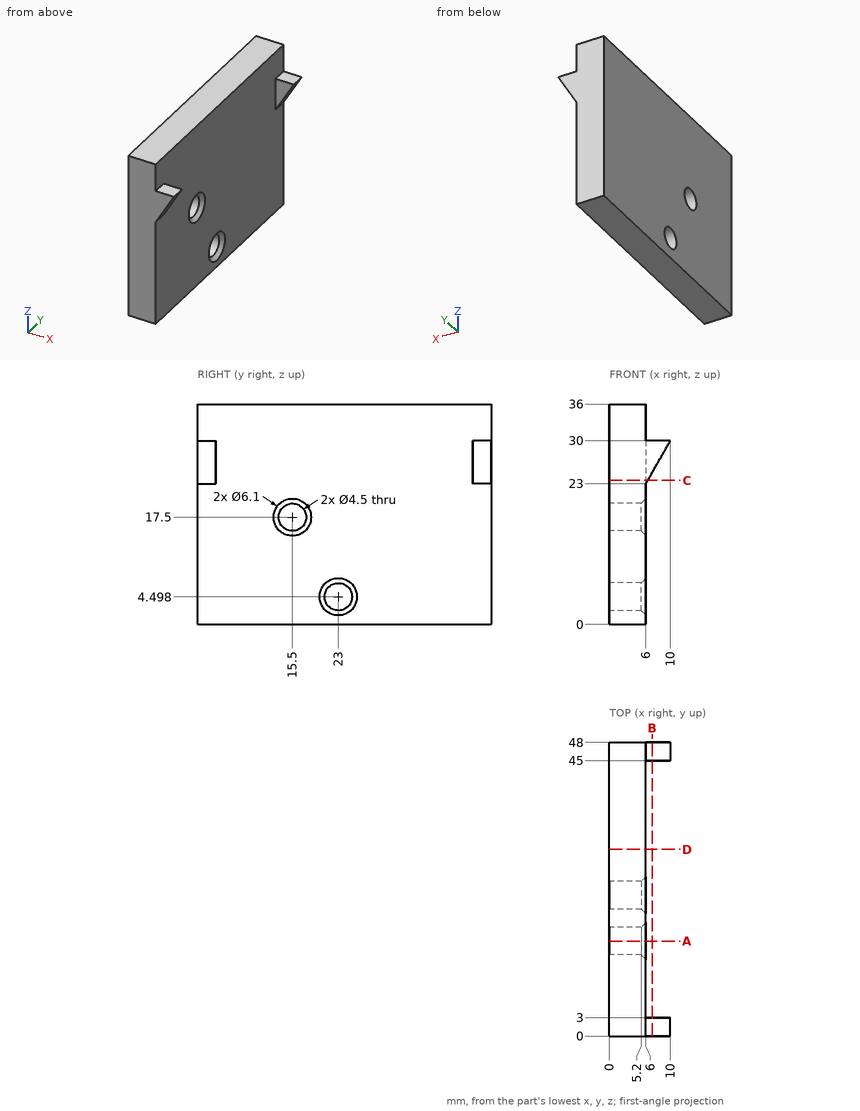
Input: dimensioned drawing with shaded views. Units: mm. Origin: part minimum x, y, z. Give positions to 0.01 mm unless a question says otherwise; leave off trailing zeros. Loops run counter-clockwise (first coordinate to the right, second up) from the corner with the lowest first, then second, coordinate; pieces in that order, holes last. Notation, with made-up numbers: (2.5, 26) -> (16.5, 26) arc R24 cw to (16.5, 54) -> close; hole circle Ø8 at (78.5, 4). An arc over 180 degrees is marked (long way). Use a Markdown table: item, result. Add a question column.
1) First-contact query: pin 1 (11 mm diameter, centred on y = 34, z = 21, fed in from +X); pin 2 (5 mm diameter, centred on x = 9, y = 8.5, fed in from +Z); pin 3 (0.9 mm diameter, centred on x = 7, y = 2, fed in from +Z). Flat tips, straight axial feed; report the tip coordinate or a pass-through.
2) Line query: line 1 along Z through (x, y) = (3.25, 23); line 2 along Y through (x, z) = (2.7, 17.5); line 3 along X through (y, z) = (32, 11). Output: solid intervals per line, ascending. Write a range as [from, to].
3) Section query B-B, the plane x = 7. Return the cut outline in (y, z).
4) Section query A-A, the plane y = 15.5. Return the cut outline in (x, z), then the cut area to 3 significant figures.
5) Section query D-D, the plane y = 30.5. Return the cut outline in (x, z), then the cut area to 3 significant figures.
6) Section query C-C, the plane z = 23.5. Return the cut outline in (x, y).
Numbers:
| question | item | result |
|---|---|---|
| 1 | pin 1 | stops at x = 6 |
| 1 | pin 2 | passes through |
| 1 | pin 3 | stops at z = 30 |
| 2 | line 1 | z = [0, 2.25], [6.75, 36] |
| 2 | line 2 | y = [0, 13.25], [17.75, 48] |
| 2 | line 3 | x = [0, 6] |
| 3 | outline | (0, 24.75) -> (3, 24.75) -> (3, 30) -> (0, 30) -> close; (45, 24.75) -> (48, 24.75) -> (48, 30) -> (45, 30) -> close |
| 4 | outline | (0, 0) -> (6, 0) -> (6, 14.45) -> (5.2, 15.25) -> (0, 15.25) -> close; (0, 19.75) -> (5.2, 19.75) -> (6, 20.55) -> (6, 36) -> (0, 36) -> close |
| 4 | area | 188 mm2 |
| 5 | outline | (0, 0) -> (6, 0) -> (6, 36) -> (0, 36) -> close |
| 5 | area | 216 mm2 |
| 6 | outline | (0, 0) -> (6.29, 0) -> (6.29, 3) -> (6, 3) -> (6, 45) -> (6.29, 45) -> (6.29, 48) -> (0, 48) -> close |
